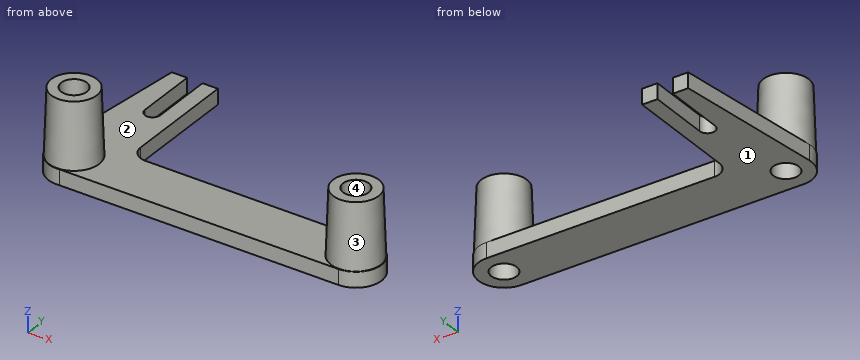
```python
from build123d import *

# Parameters (mm, degrees)
BASE_EXTRUSION_DEPTH         = 3
ESQUISSE3_R                  = 4.999999999999999
BOSS_EXTRU_1_DEPTH           = 15.8
BOSS_EXTRU_1_DRAFT           = -2.0000000000000044
ESQUISSE3_R_2                = 4.9999999999999964
BOSS_EXTRU_1_PROFILE_2_DEPTH = 15.8
BOSS_EXTRU_1_PROFILE_2_DRAFT = -2.0000000000000044
PER_AGE1_D                   = 5
PER_AGE1_DEPTH               = 15.8
PER_AGE1_TIP                 = 1.5021515475689007
PER_AGE3_D                   = 5
PER_AGE3_DEPTH               = 15.8
PER_AGE3_TIP                 = 1.5021515475689007


with BuildPart() as part:
    # Esquisse1 → Base-Extrusion (new body)
    with BuildSketch(Plane.XY):
        with BuildLine():
            Line((0.6787939241914508, -3.1163780736354636), (55.149951438834705, -3.116378073635477))
            ThreePointArc((55.149951438834705, -3.116378073635477), (60.149951438834705, 1.883621926364523), (55.149951438834705, 6.883621926364523))
            Line((55.149951438834705, 6.883621926364523), (10.649951438834709, 6.883621926364541))
            ThreePointArc((10.649951438834709, 6.883621926364541), (8.528631095275069, 7.7623015828049), (7.649951438834709, 9.88362192636454))
            Line((7.649951438834709, 9.88362192636454), (7.649951438834716, 31.855575830583856))
            Line((7.649951438834716, 31.855575830583856), (4.649951438834716, 31.855575830583856))
            Line((4.649951438834716, 31.855575830583856), (4.649951438834713, 19.855575830583852))
            ThreePointArc((4.649951438834713, 19.855575830583852), (3.149951438834714, 18.355575830583852), (1.6499514388347154, 19.855575830583852))
            Line((1.6499514388347154, 19.855575830583852), (1.6499514388347158, 31.85557583058385))
            Line((1.6499514388347158, 31.85557583058385), (-1.350048561165284, 31.855575830583856))
            Line((-1.350048561165284, 31.855575830583856), (-4.815702167023938, 2.440626483624255))
            ThreePointArc((-4.815702167023938, 2.440626483624255), (-3.4055229517499925, -1.6599044862286791), (0.6787939241914508, -3.1163780736354636))
        make_face()
    extrude(amount=BASE_EXTRUSION_DEPTH)


with BuildPart() as boss_extru_1_tool:
    # Esquisse3 → Boss.-Extru.1 (with draft: the straight prism first)
    with BuildSketch(Plane(origin=(0, 0, 0), x_dir=(-1, 0, 0), z_dir=(0, 0, -1))):
        with Locations((-0.1499514388347119, 1.8555758305838532)):
            Circle(ESQUISSE3_R)
    extrude(amount=-BOSS_EXTRU_1_DEPTH)
    # Boss.-Extru.1: the draft: its side faces are tilted about the plane it starts from
    boss_extru_1_sides = [boss_extru_1_tool.faces().sort_by_distance(p)[0] for p in [
        (5.149951439, 1.855575831, 7.9),
    ]]
    draft(boss_extru_1_sides, Plane(origin=(0, 0, 0), x_dir=(-1, 0, 0), z_dir=(0, 0, -1)), BOSS_EXTRU_1_DRAFT)


with BuildPart() as part_1:
    add(part.part)

    # Boss.-Extru.1: add boss_extru_1_tool
    add(boss_extru_1_tool.part)


with BuildPart() as boss_extru_1_profile_2_tool:
    # Esquisse3 → Boss.-Extru.1 profile 2 (with draft: the straight prism first)
    with BuildSketch(Plane(origin=(0, 0, 0), x_dir=(-1, 0, 0), z_dir=(0, 0, -1))):
        with Locations((-55.149951438834705, 1.883621926364523)):
            Circle(ESQUISSE3_R_2)
    extrude(amount=-BOSS_EXTRU_1_PROFILE_2_DEPTH)
    # Boss.-Extru.1 profile 2: the draft: its side faces are tilted about the plane it starts from
    boss_extru_1_profile_2_sides = [boss_extru_1_profile_2_tool.faces().sort_by_distance(p)[0] for p in [
        (60.149951439, 1.883621926, 7.9),
    ]]
    draft(boss_extru_1_profile_2_sides, Plane(origin=(0, 0, 0), x_dir=(-1, 0, 0), z_dir=(0, 0, -1)), BOSS_EXTRU_1_PROFILE_2_DRAFT)


with BuildPart() as part_2:
    add(part_1.part)

    # Boss.-Extru.1 profile 2: add boss_extru_1_profile_2_tool
    add(boss_extru_1_profile_2_tool.part)

    # Perçage1
    with Locations(Plane.XY.offset(15.8)):
        with Locations((55.149951439, 1.883621926)):
            Hole(PER_AGE1_D / 2, depth=PER_AGE1_DEPTH)
            with Locations((0, 0, -(PER_AGE1_DEPTH + PER_AGE1_TIP / 2))):  # 118° drill point
                Cone(0, PER_AGE1_D / 2, PER_AGE1_TIP, mode=Mode.SUBTRACT)

    # Perçage3
    with Locations(Plane.XY.offset(15.8)):
        with Locations((0.149951439, 1.855575831)):
            Hole(PER_AGE3_D / 2, depth=PER_AGE3_DEPTH)
            with Locations((0, 0, -(PER_AGE3_DEPTH + PER_AGE3_TIP / 2))):  # 118° drill point
                Cone(0, PER_AGE3_D / 2, PER_AGE3_TIP, mode=Mode.SUBTRACT)


solid = part_2.part
```
The model under review builds one solid part; all positions refer to its coordinate system, in mm. Face numbers are marked on the shaded views. A direction names the side the tool comes from. Round coordinates to 2 decimals unless told otherwise and drop trailing zeros. Order: outer loops, then holes, each group sorted by start corner. A loop starts at its lowest first (then second) coordinate and runs counter-clockwise, first axis right, second up.
(1) For P1, Ø1.5, axis at y = 23.5, z = 1.5, coming from the +X side; P2, Ø1.5, axis at x = 40.5, z = 2, coming from the -Y side; P3, Ø6.5, axis at x = 0.15, y = 1.86, coming from the +Z side; P4, Ø3, axis at x = 21.5, y = 6, coming from the +Z side, all flat-tipped, find the tip position at first contact; note any pin that passes through.
Working result:
P1: stops at x = 7.65
P2: stops at y = -3.12
P3: stops at z = 15.8
P4: stops at z = 3
(2) Take a section at C-C, the plane x = 43.5. State the section outline as (y, z) points, plus the area to 3 significant figures.
Working result:
outline: (-3.12, 0) - (6.88, 0) - (6.88, 3) - (-3.12, 3) - close
area: 30.0 mm2
(3) Tool access review of the marked faces 3 and 4: name each direction out of +Z, -Z, +X, -X, +Y, -Y from which nothing blocks a thin tool from reaching the whole face with its end or side.
Working result:
face 3: +Z
face 4: +Z, -Z
(4) Take a section at D-D, the plane y = 25. State the section outline as (x, z) points.
Working result:
outline: (-2.16, 0) - (1.65, 0) - (1.65, 3) - (-2.16, 3) - close; (4.65, 0) - (7.65, 0) - (7.65, 3) - (4.65, 3) - close
(5) Take a section at B-B, the plane z = 9.5. State the section outline as (x, y) points, plus the area to 3 significant figures.
Working result:
outline: circle Ø9.34 at (0.15, 1.86); circle Ø9.34 at (55.15, 1.88); hole circle Ø5 at (0.15, 1.86); hole circle Ø5 at (55.15, 1.88)
area: 97.7 mm2
(6) Take a section at A-A, the plane y = 20.5. State the section outline as (x, z) points, plus the area to 3 significant figures.
Working result:
outline: (-2.69, 0) - (1.65, 0) - (1.65, 3) - (-2.69, 3) - close; (4.65, 0) - (7.65, 0) - (7.65, 3) - (4.65, 3) - close
area: 22.0 mm2
(7) Wall thickness on L1, parallel to X at y = 2, z = 2; L2, parallel to Z at x = 25.5, y = -2; L3, parallel to X at y = 29, z = 1: over which ranges is each line inside the solid? List them lowest first.
Working result:
L1: x = -4.85 to -2.35, 2.65 to 52.65, 57.65 to 60.15
L2: z = 0 to 3
L3: x = -1.69 to 1.65, 4.65 to 7.65
(8) Mouldability with a two-part tool opening along X and no side actions: class the marked faces 1 and 2 as released by +X, released by -X, zero draft, split by the parting line, or undercut.
Working result:
face 1: zero draft
face 2: undercut
